Input: part model. Units: mm. Frame: model coordinates. A direction names the side the tool comes from. Round coordinates to 2 decimals unless told otherwise and drop trailing zeros. Order: outer loops, then holes, each group sorted by start corner. A loop starts at its lowest first (then second) coordinate and runs counter-clockwise, first axis right, second up. Notation, with made-up numbers: (56.5, 52.25) - (103.5, 52.25) arc R16 cw to (103.5, 76.25) - close; hole circle Ø2 at (-28.5, 69). An arc over 180 degrees is marked (long way). One line per item, written item: value. Start each with the question number.
from build123d import *

# Parameters (mm, degrees)
F0_R     = 1.496924
F0_R_2   = 3.477607
F0_R_3   = 5.000213
F0_R_4   = 5.256627
F0_R_5   = 4.304855
F0_R_6   = 4.385843
F0_R_7   = 3.153201
F0_R_8   = 5.870011
F0_R_9   = 1.567334
F0_R_10  = 4.321853
F0_R_11  = 5.459754
F1_DEPTH = 12.7
F0_R_12  = 7.190762
F0_R_13  = 5.715
F2_DEPTH = 7.62
F3_DEPTH = 12.7


with BuildPart() as f1:
    # F0 (on Top) → F1 (new body)
    with BuildSketch(Plane.XY):
        with BuildLine():
            Line((-131.803075, 61.526629), (-132.53006, 17.42161))
            add(Edge.make_bspline(
                [(-132.53006, 17.42161), (-132.53006, 16.438883), (-150.375057, 16.976569), (-151.139576, 7.47687)],
                knots=[0, 0, 0, 0, 21.100047, 21.100047, 21.100047, 21.100047], degree=3))
            Line((-151.139576, 7.47687), (-150.796539, -89.187486))
            add(Edge.make_bspline(
                [(-150.796539, -89.187486), (-149.725936, -97.980395), (-143.849122, -101.201955), (-136.357958, -101.974052)],
                knots=[0, 0, 0, 0, 19.286496, 19.286496, 19.286496, 19.286496], degree=3))
            Line((-136.357958, -101.974052), (-135.276752, -101.974052))
            Line((-135.276752, -101.974052), (-101.682383, -103.054997))
            Line((-101.682383, -103.054997), (-101.712527, -103.991822))
            Line((-101.712527, -103.991822), (-87.849766, -103.991822))
            Line((-87.849766, -103.991822), (-87.858493, -102.977792))
            Line((-87.858493, -102.977792), (-51.757253, -101.539352))
            add(Edge.make_bspline(
                [(-38.531929, -89.229472), (-40.675483, -99.353819), (-46.844892, -101.366516), (-51.757253, -101.539352)],
                knots=[0, 0, 0, 0, 18.067715, 18.067715, 18.067715, 18.067715], degree=3))
            Line((-38.531929, -89.229472), (-38.531929, 7.680066))
            add(Edge.make_bspline(
                [(-57.082368, 17.358589), (-40.642904, 13.823552), (-40.001379, 12.821936), (-38.531929, 7.680066)],
                knots=[0, 0, 0, 0, 20.923494, 20.923494, 20.923494, 20.923494], degree=3))
            Line((-57.082368, 17.358589), (-57.757391, 61.679844))
            add(Edge.make_bspline(
                [(-57.757391, 61.679844), (-58.758005, 63.463514), (-60.22691, 70.734918), (-69.454086, 72.549358)],
                knots=[0, 0, 0, 0, 15.967435, 15.967435, 15.967435, 15.967435], degree=3))
            add(Edge.make_bspline(
                [(-119.06031, 72.685671), (-98.531029, 75.251681), (-82.806464, 74.541935), (-69.454086, 72.549358)],
                knots=[0, 0, 0, 0, 49.606411, 49.606411, 49.606411, 49.606411], degree=3))
            add(Edge.make_bspline(
                [(-131.803075, 61.526629), (-128.101333, 71.713794), (-122.839052, 71.691977), (-119.06031, 72.685671)],
                knots=[0, 0, 0, 0, 16.93819, 16.93819, 16.93819, 16.93819], degree=3))
        make_face()
        with Locations((-125.477582, -39.376188)):
            Circle(F0_R, mode=Mode.SUBTRACT)
        with Locations((-117.514238, -57.91628)):
            Circle(F0_R_2, mode=Mode.SUBTRACT)
        with Locations((-117.421836, -19.4379)):
            Circle(F0_R_3, mode=Mode.SUBTRACT)
        with BuildLine():
            add(Edge.make_bspline(
                [(-92.559412, -2.722392), (-99.928118, -11.216616), (-120.820127, -30.964935), (-108.078144, -47.028057)],
                knots=[0, 0, 0, 0, 46.944894, 46.944894, 46.944894, 46.944894], degree=3))
            Line((-92.559412, -2.722392), (-79.016782, -7.556637))
            add(Edge.make_bspline(
                [(-79.016782, -7.556637), (-83.614662, -11.021999), (-88.109598, -15.379434), (-91.712408, -19.805491)],
                knots=[0, 0, 0, 0, 17.64124, 17.64124, 17.64124, 17.64124], degree=3))
            add(Edge.make_bspline(
                [(-91.712408, -19.805491), (-71.812876, -19.32627), (-73.281839, -42.991612), (-78.178406, -46.745423)],
                knots=[0, 0, 0, 0, 30.148452, 30.148452, 30.148452, 30.148452], degree=3))
            add(Edge.make_bspline(
                [(-108.078144, -47.028057), (-100.131333, -56.782793), (-82.993366, -54.98749), (-78.178406, -46.745423)],
                knots=[0, 0, 0, 0, 29.901075, 29.901075, 29.901075, 29.901075], degree=3))
        make_face(mode=Mode.SUBTRACT)
        with Locations((-89.558132, -64.366221)):
            Circle(F0_R_4, mode=Mode.SUBTRACT)
        with Locations((-64.769246, -30.964935)):
            Circle(F0_R_5, mode=Mode.SUBTRACT)
        with Locations((-133.611128, -11.011187)):
            Circle(F0_R_6, mode=Mode.SUBTRACT)
        with Locations((-108.078144, -7.924549)):
            Circle(F0_R_7, mode=Mode.SUBTRACT)
        with Locations((-95.0303, 63.422114)):
            Circle(F0_R_8, mode=Mode.SUBTRACT)
        with Locations((-69.72374, -11.021999)):
            Circle(F0_R_9, mode=Mode.SUBTRACT)
        with Locations((-68.831384, 7.891561)):
            Circle(F0_R_10, mode=Mode.SUBTRACT)
        with Locations((-88.109598, 9.438152)):
            Circle(F0_R_11, mode=Mode.SUBTRACT)
        Polygon((-127.203408, 20.682184), (-127.325644, 52.755584), (-61.360919, 52.755584), (-61.360919, 20.682184), align=None, mode=Mode.SUBTRACT)
        with BuildLine():
            Line((-79.016782, -7.556637), (-92.559412, -2.722392))
            add(Edge.make_bspline(
                [(-92.559412, -2.722392), (-99.928118, -11.216616), (-120.820127, -30.964935), (-108.078144, -47.028057)],
                knots=[0, 0, 0, 0, 46.944894, 46.944894, 46.944894, 46.944894], degree=3))
            add(Edge.make_bspline(
                [(-108.078144, -47.028057), (-100.131333, -56.782793), (-82.993366, -54.98749), (-78.178406, -46.745423)],
                knots=[0, 0, 0, 0, 29.901075, 29.901075, 29.901075, 29.901075], degree=3))
            add(Edge.make_bspline(
                [(-91.712408, -19.805491), (-71.812876, -19.32627), (-73.281839, -42.991612), (-78.178406, -46.745423)],
                knots=[0, 0, 0, 0, 30.148452, 30.148452, 30.148452, 30.148452], degree=3))
            add(Edge.make_bspline(
                [(-79.016782, -7.556637), (-83.614662, -11.021999), (-88.109598, -15.379434), (-91.712408, -19.805491)],
                knots=[0, 0, 0, 0, 17.64124, 17.64124, 17.64124, 17.64124], degree=3))
        make_face()
        with BuildLine():
            add(Edge.make_bspline(
                [(-92.559412, -4.335725), (-105.420828, -19.4379), (-113.935962, -30.403955), (-108.555153, -43.363504)],
                knots=[0, 0, 0, 0, 42.178564, 42.178564, 42.178564, 42.178564], degree=3))
            Line((-92.559412, -4.335725), (-82.505698, -7.924549))
            add(Edge.make_bspline(
                [(-82.505698, -7.924549), (-87.019771, -12.31665), (-91.893606, -16.58126), (-95.404953, -22.153838)],
                knots=[0, 0, 0, 0, 19.205817, 19.205817, 19.205817, 19.205817], degree=3))
            add(Edge.make_bspline(
                [(-95.404953, -22.153838), (-80.268763, -17.979054), (-75.162396, -31.588022), (-77.190861, -41.397225)],
                knots=[0, 0, 0, 0, 26.496436, 26.496436, 26.496436, 26.496436], degree=3))
            add(Edge.make_bspline(
                [(-108.555153, -43.363504), (-102.122009, -55.195887), (-84.086247, -55.540521), (-77.190861, -41.397225)],
                knots=[0, 0, 0, 0, 31.425866, 31.425866, 31.425866, 31.425866], degree=3))
        make_face(mode=Mode.SUBTRACT)
        Polygon((-61.360919, 52.755584), (-127.325644, 52.755584), (-127.203408, 20.682184), (-61.360919, 20.682184), align=None)
        Polygon((-67.204248, 26.135962), (-121.871863, 26.135962), (-121.612164, 47.301807), (-67.204248, 47.301807), align=None, mode=Mode.SUBTRACT)
        Polygon((-121.612164, 47.301807), (-121.871863, 26.135962), (-67.204248, 26.135962), (-67.204248, 47.301807), align=None)
        Polygon((-68.156406, 27.233338), (-120.712638, 27.233338), (-120.479164, 46.26181), (-68.156406, 46.403773), align=None, mode=Mode.SUBTRACT)
    extrude(amount=F1_DEPTH)

    # F0 (on Top) → F2 (join)
    with BuildSketch(Plane.XY):
        with Locations((-88.109598, 9.438152)):
            Circle(F0_R_11)
        with Locations((-68.831384, 7.891561)):
            Circle(F0_R_10)
        with Locations((-69.72374, -11.021999)):
            Circle(F0_R_9)
        with Locations((-64.769246, -30.964935)):
            Circle(F0_R_5)
        with Locations((-108.078144, -7.924549)):
            Circle(F0_R_7)
        with Locations((-117.421836, -19.4379)):
            Circle(F0_R_3)
        with Locations((-133.611128, -11.011187)):
            Circle(F0_R_6)
        with Locations((-125.477582, -39.376188)):
            Circle(F0_R)
        with Locations((-117.514238, -57.91628)):
            Circle(F0_R_2)
        with Locations((-89.558132, -64.366221)):
            Circle(F0_R_4)
        with BuildLine():
            Line((-82.505698, -7.924549), (-92.559412, -4.335725))
            add(Edge.make_bspline(
                [(-92.559412, -4.335725), (-105.420828, -19.4379), (-113.935962, -30.403955), (-108.555153, -43.363504)],
                knots=[0, 0, 0, 0, 42.178564, 42.178564, 42.178564, 42.178564], degree=3))
            add(Edge.make_bspline(
                [(-108.555153, -43.363504), (-102.122009, -55.195887), (-84.086247, -55.540521), (-77.190861, -41.397225)],
                knots=[0, 0, 0, 0, 31.425866, 31.425866, 31.425866, 31.425866], degree=3))
            add(Edge.make_bspline(
                [(-95.404953, -22.153838), (-80.268763, -17.979054), (-75.162396, -31.588022), (-77.190861, -41.397225)],
                knots=[0, 0, 0, 0, 26.496436, 26.496436, 26.496436, 26.496436], degree=3))
            add(Edge.make_bspline(
                [(-82.505698, -7.924549), (-87.019771, -12.31665), (-91.893606, -16.58126), (-95.404953, -22.153838)],
                knots=[0, 0, 0, 0, 19.205817, 19.205817, 19.205817, 19.205817], degree=3))
        make_face()
        with Locations((-93.40658, -36.362156)):
            Circle(F0_R_12, mode=Mode.SUBTRACT)
        Polygon((-120.479164, 46.26181), (-120.712638, 27.233338), (-68.156406, 27.233338), (-68.156406, 46.403773), align=None)
        with Locations((-93.40658, -36.362156)):
            Circle(F0_R_13)
        with Locations((-93.40658, -36.362156)):
            Circle(F0_R_12)
        with Locations((-93.40658, -36.362156)):
            Circle(F0_R_13, mode=Mode.SUBTRACT)
    extrude(amount=F2_DEPTH)

    # F0 (on Top) → F3 (join)
    with BuildSketch(Plane.XY):
        with Locations((-93.40658, -36.362156)):
            Circle(F0_R_13)
    extrude(amount=F3_DEPTH)


solid = f1.part
1. Line query: line 1 (Z direction, x = -88, y = -32.5); line 2 (X direction, y = -10, z = 9); line 3 (Y direction, x = -82, z = 10.5). Output: solid intervals per line, ascending. Write a range as from..to.
2. Section A-A (y = 35.5). Return the cut outline in (x, z), then the cut area to 3 significant figures.
3. Set-up query: faces 1 (the face through (-70.06, -102.27, 6.26)), 2 (the face through (-87.955, -34.646, 10.124)). Return all of +Z, -Z, +X, -X, +Y, -Y with unobstructed straight access to the full face (end or side cutting, diameter ignored); none if empty.
4. Pin query (flat end, axial travel): pin 1 (2.5 mm diameter, centred on x = -65.5, y = -30.5, fed in from +Z); pin 2 (1 mm diameter, centred on x = -119, z = 3.5, fed in from +Y); pin 3 (3 mm diameter, centred on x = -116, z = 9.5, fed in from -Y). Return the tip coordinate at first contact, or that it passes through.
5. Section C-C (y = 53.5). Return the cut outline in (x, z).
6. Pull-direction query (Y, two-part tool) for faces 3 (the face through (-93, -36, 12.7)), 4 (the face through (-69, 8, 7.62)), 5 (the face through (-95, -103.992, 6)); classes: released by +Y, released by -Y, zero draft, split by the parting line, or undercut.
7. Section B-B (z = 10.75). State how many separate pieces and enclosed holes the cut face has, then the cut area to 3 significant figures.
Solved:
1. line 1: z = 0..7.62
1. line 2: x = -151.08..-137.88, -129.34..-110.45, -105.7..-97.31, -84.66..-70.91, -68.54..-38.53
1. line 3: y = -102.74..-47.76, -24.19..27.23, 46.37..73.93
2. outline: (-132.23, 0) - (-57.36, 0) - (-57.36, 12.7) - (-68.16, 12.7) - (-68.16, 7.62) - (-120.61, 7.62) - (-120.61, 12.7) - (-132.23, 12.7) - close
2. area: 684 mm²
3. face 1: +Z, -Z, +X, -Y
3. face 2: +Z
4. pin 1: stops at z = 7.62
4. pin 2: stops at y = 72.76
4. pin 3: stops at y = -102.64
5. outline: (-131.94, 0) - (-57.63, 0) - (-57.63, 12.7) - (-131.94, 12.7) - close
6. face 3: zero draft
6. face 4: undercut
6. face 5: released by -Y
7. separate pieces: 2
7. enclosed holes: 13
7. area: 14,800 mm²
